from build123d import *

# Parameters (mm, degrees)
EXTRUDE_1_DEPTH     = 6
SKETCH_4_R          = 2
SKETCH_4_R_2        = 4
CUT_EXTRUDE_2_DEPTH = 80.630396206
M3X0_5_1_REACH      = 81.63
M3X0_5_1_BORE_R     = 1.25
CHAMFER_1_SIZE      = 1


with BuildPart() as part:
    # ｽｹｯﾁ3 → ﾎﾞｽ - 押し出し1 (new body)
    with BuildSketch(Plane.XY):
        Polygon((0, -47), (0, 47), (14, 47), (14, 7), (64, 7), (64, -7), (14, -7), (14, -47), align=None)
    extrude(amount=EXTRUDE_1_DEPTH)

    # ｽｹｯﾁ4 → ｶｯﾄ - 押し出し2 (cut, through all)
    with BuildSketch(Plane.XY.offset(6)):
        with Locations((7, 40)):
            Circle(SKETCH_4_R)
        with Locations((7, -40)):
            Circle(SKETCH_4_R)
        with Locations((7, 0)):
            Circle(SKETCH_4_R)
        with Locations((57, 0)):
            Circle(SKETCH_4_R_2)
    extrude(amount=-CUT_EXTRUDE_2_DEPTH, mode=Mode.SUBTRACT)

    # M3x0.5 ねじ穴1 bore → M3x0.5 ねじ穴1 (cut, up to next)
    with BuildSketch(Plane.ZY, mode=Mode.PRIVATE) as m3x0_5_1_sk1:
        with Locations((3, -40)):
            Circle(M3X0_5_1_BORE_R)
    m3x0_5_1_tool1 = extrude(m3x0_5_1_sk1.sketch, amount=-M3X0_5_1_REACH, mode=Mode.PRIVATE) & part.part
    # M3x0.5 ねじ穴1 bore → M3x0.5 ねじ穴1 (cut, up to next)
    with BuildSketch(Plane.ZY, mode=Mode.PRIVATE) as m3x0_5_1_sk2:
        with Locations((3, 40)):
            Circle(M3X0_5_1_BORE_R)
    m3x0_5_1_tool2 = extrude(m3x0_5_1_sk2.sketch, amount=-M3X0_5_1_REACH, mode=Mode.PRIVATE) & part.part
    # M3x0.5 ねじ穴1 bore → M3x0.5 ねじ穴1 (cut, up to next)
    with BuildSketch(Plane.ZY, mode=Mode.PRIVATE) as m3x0_5_1_sk3:
        with Locations((3, 0)):
            Circle(M3X0_5_1_BORE_R)
    m3x0_5_1_tool3 = extrude(m3x0_5_1_sk3.sketch, amount=-M3X0_5_1_REACH, mode=Mode.PRIVATE) & part.part
    add(m3x0_5_1_tool1.solids().sort_by_distance((0, -40, 3))[0], mode=Mode.SUBTRACT)
    add(m3x0_5_1_tool2.solids().sort_by_distance((0, 40, 3))[0], mode=Mode.SUBTRACT)
    add(m3x0_5_1_tool3.solids().sort_by_distance((0, 0, 3))[0], mode=Mode.SUBTRACT)

    # 面取り1
    chamfer_1_edges = [part.edges().sort_by_distance(p)[0] for p in [
        (64, 7, 3),
        (64, -7, 3),
        (14, -47, 3),
        (0, -47, 3),
        (0, 47, 3),
        (14, 47, 3),
    ]]
    chamfer(chamfer_1_edges, length=CHAMFER_1_SIZE)


solid = part.part
Could you check a few things on this model? Use its own coordinates, in mm. A direction names the side the tool comes from. Coordinates: 2 decimals unless noted, no trailing zeros. Order: outer loops, then holes, each group sorted by start corner. A loop starts at its lowest first (then second) coordinate and runs counter-clockwise, first axis right, second up. Notation, with made-up numbers: (-32, 6) -> (0, 6) arc R33 cw to (0, 41) -> close; hole circle Ø10 at (32, 49). An arc over 180 degrees is marked (long way). One line per question, with ' | ' between items.
Q1. On a 3-axis mill with a long thin cutter (end or side, diameter ignored), from which of +Z, -Z, +X, -X, +Y, -Y can I reach the whole of each face in a straight line? I mean faces 5 (the face through (60.815, 1.201, 3.042)), 6 (the face through (38, 7, 3)), 7 (the face through (14, -26, 3)), 8 (the face through (64, 0, 3)), 9 (the face through (2.68, -39.95, 1.75)). Say none if no direction works.
Return value:
face 5: +Z, -Z | face 6: +Z, -Z, +X, +Y | face 7: +Z, -Z, +X, -Y | face 8: +Z, -Z, +X, +Y, -Y | face 9: -X
Q2. I'm going to push flat-ended pins straight in: P1, Ø1.8, axis at y = -36, z = 1.5, coming from the +X side; P2, Ø3, axis at x = 41, z = 3, coming from the -Y side; P3, Ø1.5, axis at y = 40, z = 3, coming from the -X side. Where does each tip first touch, or does it pass through?
Return value:
P1: x = 14 | P2: y = -7 | P3: x = 8.85
Q3. If I drill on L1, parallel to Y at x = 7, z = 2.5; L2, parallel to Y at x = 2.55, z = 3; L3, parallel to Z at x = 1, y = -40, over which ranges is the centre line in solid material (lowest first)?
Return value:
L1: -47 to -42, -38 to -2, 2 to 38, 42 to 47 | L2: -47 to -41.25, -38.75 to -1.25, 1.25 to 38.75, 41.25 to 47 | L3: 0 to 1.75, 4.25 to 6
Q4. Imagine slicing it at C-C on y = -40. Please give me the cut outline in (x, z), and give its area (3 significant figures).
Return value:
outline: (0, 0) -> (5, 0) -> (5, 1.75) -> (0, 1.75) -> close; (0, 4.25) -> (5, 4.25) -> (5, 6) -> (0, 6) -> close; (9, 0) -> (14, 0) -> (14, 6) -> (9, 6) -> close | area: 47.5 mm²
Q5. Imagine slicing it at D-D on x = 7. Please give me the cut outline in (y, z), and give its area (3 significant figures).
Return value:
outline: (-47, 0) -> (-42, 0) -> (-42, 6) -> (-47, 6) -> close; (-38, 0) -> (-2, 0) -> (-2, 6) -> (-38, 6) -> close; (2, 0) -> (38, 0) -> (38, 6) -> (2, 6) -> close; (42, 0) -> (47, 0) -> (47, 6) -> (42, 6) -> close | area: 492 mm²
Q6. Thinking about a two-plate mould opening in X: for faces 1 (the face through (39, -7, 3)), 2 (the face through (14, 27, 3)), 3 (the face through (8.908, 40.601, 3.042)), 4 (the face through (0, -1, 2)), which applies, pulls with the +X half, pulls with the -X half, needs draft (parallel to the pull), parting line crosses it, or undercut?
Return value:
face 1: needs draft | face 2: pulls with the +X half | face 3: undercut | face 4: pulls with the -X half
Q7. Imagine slicing it at A-A on x = 57. Please give me the cut outline in (y, z), and give its area (3 significant figures).
Return value:
outline: (-7, 0) -> (-4, 0) -> (-4, 6) -> (-7, 6) -> close; (4, 0) -> (7, 0) -> (7, 6) -> (4, 6) -> close | area: 36.0 mm²
Q8. Imagine slicing it at B-B on z = 3. Please give me the cut outline in (x, y).
Return value:
outline: (0, -46) -> (1, -47) -> (13, -47) -> (14, -46) -> (14, -7) -> (63, -7) -> (64, -6) -> (64, 6) -> (63, 7) -> (14, 7) -> (14, 46) -> (13, 47) -> (1, 47) -> (0, 46) -> (0, 41.25) -> (5.44, 41.25) arc R2 cw (long way) to (5.44, 38.75) -> (0, 38.75) -> (0, 1.25) -> (5.44, 1.25) arc R2 cw (long way) to (5.44, -1.25) -> (0, -1.25) -> (0, -38.75) -> (5.44, -38.75) arc R2 cw (long way) to (5.44, -41.25) -> (0, -41.25) -> close; hole circle Ø8 at (57, 0)
